Here's how the part is built. I have some questions about the finished solid (model axes, mm). A direction names the side the tool comes from. Coordinates: 2 decimals unless noted, no trailing zeros. Write each loop counter-clockwise with the first axis right and the second up, starting at its lowest first coordinate (ties: lowest second). Pieces come first, ordered by that corner, then holes. Notation, with made-up numbers: M 62,16.5 L 98,16.5 A22 ccw 98,22.5 Z; hole C 24,-30 d7. An arc over 180 degrees is marked long. Use one line per item in the form item = value. Start each with the question number.
1. On a 3-axis mill with a long thin cutter (end or side, diameter ignored), from which of +Z, -Z, +X, -X, +Y, -Y can I reach the whole of each face in a straight line? I mean faces 4 (the face through (0, 2, 26)), 5 (the face through (28, 3.2, -20)). Say none if no direction works.
2. I want a section at C-C, the plane z = 0. List the corners of the cut face in (x, y) for me, plus the area to 3 significant figures.
3. I want a section at D-D, the plane x = 19.5. List the corners of the cut face in (y, z) for me, plus the area to 3 significant figures.
4. Thinking about a two-plate mould opening in Z: for faces 1 (the face through (29, 2, -43)), 2 (the face through (-31.636, 1.578, 0.215)), 3 (the face through (28, 0, -20)), which applies, released by +Z, released by -Z, zero draft, split by the parting line, or undercut?
5. I want a section at A-A, the plane z = -35. List the corners of the cut face in (x, y) for me.
6. I'm going to push a flat-ended pin straight in: pin 1 Ø4 at (x, z) = (53.47, 35) entering from -Y. Where does the tip first touch, or does it pass through?
7. Please list where these lines run through material, in increasing order: line 1 along X through (y, z) = (1.55, 0); line 2 along X through (y, z) = (2.65, -1); line 3 along Z through (x, y) = (0.5, 0.25). Write a range as [from, to].
8. I want a section at B-B, the plane x = 53.47. List the corners of the cut face in (y, z) for me, plus the area to 3 significant figures.
from build123d import *

# Parameters (mm, degrees)
SKETCH1_R           = 1.65
BOSS_EXTRUDE1_DEPTH = 3.2
FILLET1_R           = 10


with BuildPart() as part:
    # Sketch1 → Boss-Extrude1 (new body)
    with BuildSketch(Plane(origin=(0, 0, 0), x_dir=(1, 0, 0), z_dir=(0, 1, 0))):
        with BuildLine():
            Line((0, -43), (56.67, -43))
            Line((56.67, -43), (56.67, 43))
            Line((56.67, 43), (0, 43))
            ThreePointArc((0, 43), (-43, 0), (0, -43))
        make_face()
        with Locations(Location((26.870057685, 26.870057685, 0), (0, 0, 270))):
            Circle(SKETCH1_R, mode=Mode.SUBTRACT)
        with Locations(Location((0, -30, 0), (0, 0, 270))):
            Circle(SKETCH1_R, mode=Mode.SUBTRACT)
        with Locations(Location((53.47, 35, 0), (0, 0, 270))):
            Circle(SKETCH1_R, mode=Mode.SUBTRACT)
        with Locations(Location((53.47, -35, 0), (0, 0, 90))):
            Circle(SKETCH1_R, mode=Mode.SUBTRACT)
        with Locations(Location((-30, 0, 0), (0, 0, 90))):
            Circle(SKETCH1_R, mode=Mode.SUBTRACT)
        with BuildLine():
            Line((-4, -32.756678708), (-4, -30))
            ThreePointArc((-4, -30), (0, -26), (4, -30))
            Line((4, -30), (4, -32.756678708))
            ThreePointArc((4, -32.756678708), (23.334523779, -23.334523779), (32.756678708, -4))
            ThreePointArc((32.756678708, -4), (33, 0), (32.756678708, 4))
            ThreePointArc((32.756678708, 4), (0, 33), (-32.756678708, 4))
            Line((-32.756678708, 4), (-30, 4))
            ThreePointArc((-30, 4), (-26, 0), (-30, -4))
            Line((-30, -4), (-32.756678708, -4))
            ThreePointArc((-32.756678708, -4), (-23.334523779, -23.334523779), (-4, -32.756678708))
        make_face(mode=Mode.SUBTRACT)
    extrude(amount=BOSS_EXTRUDE1_DEPTH)

    # Fillet1
    fillet1_edges = [part.edges().sort_by_distance(p)[0] for p in [
        (4, 1.6, 32.756678708),
        (-32.756678708, 1.6, -4),
        (-32.756678708, 1.6, 4),
        (-4, 1.6, 32.756678708),
    ]]
    fillet(fillet1_edges, radius=FILLET1_R)


solid = part.part
Answer list:
q1.face_4 = +Y, -Y
q1.face_5 = +Z, -Z, +X, -X, +Y
q2.outline = M -43,0 L -31.65,0 L -31.65,3.2 L -43,3.2 Z; M -28.35,0 L -26,0 L -26,3.2 L -28.35,3.2 Z; M 33,0 L 56.67,0 L 56.67,3.2 L 33,3.2 Z
q2.area = 120 mm²
q3.outline = M 0,-43 L 3.2,-43 L 3.2,-26.62 L 0,-26.62 Z; M 0,26.62 L 3.2,26.62 L 3.2,43 L 0,43 Z
q3.area = 105 mm²
q4.face_1 = released by -Z
q4.face_2 = undercut
q4.face_3 = zero draft
q5.outline = M -24.98,0 L 51.82,0 L 51.82,3.2 L -24.98,3.2 Z; M 55.12,0 L 56.67,0 L 56.67,3.2 L 55.12,3.2 Z
q6.pin_1 = 0
q7.line_1 = [-43, -31.65], [-28.35, -26], [33, 56.67]
q7.line_2 = [-42.99, -31.31], [-28.69, -26.13], [32.98, 56.67]
q7.line_3 = [-43, -33], [26.03, 28.43], [31.57, 43]
q8.outline = M 0,-43 L 3.2,-43 L 3.2,-36.65 L 0,-36.65 Z; M 0,-33.35 L 3.2,-33.35 L 3.2,33.35 L 0,33.35 Z; M 0,36.65 L 3.2,36.65 L 3.2,43 L 0,43 Z
q8.area = 254 mm²
